Check sheet for the modelled part. Datum: model origin and axes. Units: mm. A direction names the side the tool comes from. Round coordinates to 2 decimals unless told otherwise and drop trailing zeros. Write each loop counter-clockwise with the first axis right and the second up, starting at its lowest first coordinate (ties: lowest second). Pieces come first, ordered by that corner, then holes. Notation, with made-up numbers: (86, 7.25) -> (141, 7.25) arc R23 ccw to (141, 34.25) -> close; hole circle Ø3 at (-26.75, 71.25). An arc over 180 degrees is marked (long way). Write item = value, one per line.
Autodesk Inventor part; units mm, degrees
ref_plane "YZ Plane" through (0, 0, 0) normal (1, 0, 0) x (0, 1, 0)
ref_plane "XZ Plane" through (0, 0, 0) normal (0, 1, 0) x (-1, 0, 0)
ref_plane "XY Plane" through (0, 0, 0) normal (0, 0, 1) x (1, 0, 0)
sketch "Sketch1" plane through (0, 0, 0) normal (0, 1, 0) x (-1, 0, 0)
  line L0 (0, 0) -> (-11.1125, 0)
  line L1 (-11.1125, 0) -> (-11.1125, -334.6595)
  line L2 (-11.1125, -25.4) -> (-9.525, -25.4)
  line L3 (-9.525, -25.4) -> (-9.525, -27.178)
  line L4 (-9.525, -27.178) -> (-11.1125, -27.178)
  line L5 (0, 0) -> (0, -334.6595)
  line L6 (-11.1125, -304.8) -> (0, -304.8)
  dimension "d0" = 11.1125
  dimension "d2" = 334.6595
  dimension "d4" = 25.4
  dimension "d5" = 1.778
  dimension "d6" = 1.5875
  dimension "d7" = 304.8
revolve "Revolution1" add sketch "Sketch1" angle 360 about axis through (0, 0, 0) along (0, 0, -1) contours L5 L6 L1 L4 L3 L2 L0
properties part number "3 Piston Rod"
(1) Access from +Z, -Z, +X, -X, +Y, -Y to the whole of each face (thin tool, end or side, straight path). Record for faces 4 (the cylindrical face through (10.6, -3.34, -12.88)), 5 (the flat face through (-5, -8.3, -25.4)).
Worked answers:
face_4 = +Z, -Z
face_5 = none
(2) Material ranges on L1, parallel to Z at x = 8, y = -7.5; L2, parallel to Y at x = -0.25, z = -118.5; L3, parallel to X at y = 1, z = -43, recorded low to high. Write a range as [from, to].
Worked answers:
L1 = [-304.8, -27.18], [-25.4, 0]
L2 = [-11.11, 11.11]
L3 = [-11.07, 11.07]
(3) Sectioned sample at C-C on z = -249. Enter the section's corners in (x, y) (1 decimal), then the cut area to 3 significant figures.
Worked answers:
outline = circle Ø22.2 at (0, 0)
area = 388 mm²
(4) Sectioned sample at B-B on x = -3.75. Enter the section's corners in (y, z).
Worked answers:
outline = (-10.46, -304.8) -> (10.46, -304.8) -> (10.46, -27.18) -> (8.76, -27.18) -> (8.76, -25.4) -> (10.46, -25.4) -> (10.46, 0) -> (-10.46, 0) -> (-10.46, -25.4) -> (-8.76, -25.4) -> (-8.76, -27.18) -> (-10.46, -27.18) -> close
(5) Sectioned sample at A-A on y = 3.5. Enter the section's corners in (x, z).
Worked answers:
outline = (-10.55, -304.8) -> (10.55, -304.8) -> (10.55, -27.18) -> (8.86, -27.18) -> (8.86, -25.4) -> (10.55, -25.4) -> (10.55, 0) -> (-10.55, 0) -> (-10.55, -25.4) -> (-8.86, -25.4) -> (-8.86, -27.18) -> (-10.55, -27.18) -> close
(6) Release check for a two-part mould opening along Z. For faces 1 (the flat face through (0, 0, -304.8)), 2 (the cylindrical face through (10.6, -3.34, -167.93)), 3 (the cylindrical face through (-7.559, 5.796, -26.301)) record: pulls with the +Z half, pulls with the -Z half, needs draft (parallel to the pull), parting line crosses it, or undercut.
Worked answers:
face_1 = pulls with the -Z half
face_2 = needs draft
face_3 = undercut
(7) Go/stop test with flat-tipped pins: P1, Ø1, axis at y = -8.5, z = -172, coming from the -X side; P2, Ø5, axis at y = -2, z = -63, coming from the +X side; P3, Ø2, axis at y = 6, z = -110.5, coming from the +X side; P4, Ø5, axis at x = -3.5, z = -42, coming from the +Y side. Record where each tip stops, or that it passes through.
Worked answers:
P1 = -7.71
P2 = 11.11
P3 = 9.92
P4 = 11.07
